Autodesk Fusion 360 part; units mm, degrees
sketch "Sketch1" plane through (0, 0, 0) normal (1, 0, 0) x (0, 1, 0)
  line L0 (0, 0) -> (-230, 0)
  line L1 (-230, 0) -> (-230, 150)
  line L2 (-230, 150) -> (0, 150)
  line L3 (0, 150) -> (0, 0)
  line L4 (-230, 0) -> (-220, 0)
  line L5 (-220, 0) -> (-220, 150)
  line L6 (-220, 150) -> (-230, 150)
  line L7 (-230, 150) -> (-230, 0)
  dimension "d1" = 230
  dimension "d2" = 150
  dimension "d3" = 10
  dimension "d4" = 150
extrude "Extrude1" add sketch "Sketch1" against normal blind 10
extrude "Extrude2" add 1 faces at (-6.6667, -230, 50) along direction (0, -1, 0) blind 20
extrude "Extrude3" add 1 faces at (-6.6667, 0, 100) along direction (0, 1, 0) blind 20
sketch "Sketch2" plane through (0, 0, 0) normal (1, 0, 0) x (0, 1, 0)
  line L0 (20, 150) -> (-250, 150)
  line L1 (-250, 150) -> (-250, 0)
  line L2 (-250, 0) -> (20, 0)
  line L3 (20, 0) -> (20, 150)
  line L4 (-250, 0) -> (-240, 0)
  line L5 (-240, 0) -> (-240, 15)
  line L6 (-240, 15) -> (-250, 15)
  line L7 (-250, 15) -> (-250, 0)
  line L8 (0, 0) -> (-10, 0)
  line L9 (-10, 0) -> (-10, 15)
  line L10 (-10, 15) -> (0, 15)
  line L11 (0, 15) -> (0, 0)
  dimension "d11" = 10
  dimension "d12" = 15
  dimension "d13" = 10
  dimension "d14" = 15
  dimension "d46" = 230
extrude "Extrude12" add 1 faces at (-6.6667, -250, 50) along direction (0, -1, 0) blind 20
extrude "Extrude4" cut sketch "Sketch2" against normal blind 140 contours L1 L2 L4 L5 L6 L7 | L2 L8 L9 L10 L11
fillet "Fillet2" radius 20 1 edges at (-5, 20, 150)
sketch "Sketch3" plane through (0, 0, 0) normal (1, 0, 0) x (0, 1, 0)
  arc A0 (20, 130) -> (0, 150) centre (0, 130) ccw
  line L0 (0, 150) -> (-270, 150)
  line L1 (-250, 15) -> (-240, 15)
  line L2 (-240, 15) -> (-240, 0)
  line L3 (-270, 0) -> (-250, 0)
  line L4 (-10, 0) -> (-10, 15)
  line L5 (-10, 15) -> (0, 15)
  line L6 (0, 15) -> (0, 0)
  line L7 (0, 0) -> (20, 0)
  line L8 (20, 0) -> (20, 130)
  line L9 (-200, 0) -> (-30, 0)
  line L10 (-30, 0) -> (-30, 130)
  line L11 (-30, 130) -> (-200, 130)
  line L12 (-200, 130) -> (-200, 0)
  line L13 (-270, 150) -> (-270, 0)
  line L14 (-250, 0) -> (-250, 15)
  line L15 (-240, 0) -> (-10, 0)
extrude "Extrude5" cut sketch "Sketch3" against normal blind 100 contours L9 L10 L11 L12 L15
sketch "Sketch4" plane through (0, 0, 150) normal (0, 0, 1) x (-1, 0, 0)
  line L0 (0, 0) -> (10, 0)
  line L1 (10, 0) -> (10, 270)
  line L2 (0, 270) -> (0, 0)
  line L3 (0, 140) -> (-30, 140)
  line L4 (-30, 140) -> (-30, 111)
  line L5 (-30, 111) -> (0, 111)
  line L6 (0, 111) -> (0, 140)
  line L7 (0, 140) -> (-30, 111)
  line L8 (-30, 140) -> (0, 111)
  line L9 (-2, 138) -> (-28, 138)
  line L10 (-28, 138) -> (-28, 113)
  line L11 (-28, 113) -> (-2, 113)
  line L12 (-2, 113) -> (-2, 138)
  line L13 (-2, 138) -> (-28, 113) construction
  line L14 (-28, 138) -> (-2, 113) construction
  line L15 (10, 270) -> (0, 270)
  point P0 (-15, 125.5)
  dimension "d23" = 30
  dimension "d24" = 29
  dimension "d25" = 26
  dimension "d26" = 25
extrude "Extrude6" add sketch "Sketch4" against normal blind 10 contours L2 L6 L7 L8 L9 L11 L12 | L5 L7 L8 L11 | L3 L7 L8 L9 | L4 L7 L8 L9 L10 L11 | L7 L8 L11 | L7 L8 L9 L11 L12 | L7 L8 L9 | L7 L8 L9 L10 L11
extrude "Extrude7" cut sketch "Sketch4" against normal blind 8 contours L7 L8 L11 | L7 L8 L9 L11 L12 | L7 L8 L9 | L7 L8 L9 L10 L11
extrude "Extrude9" add 1 faces at (20, -120.6667, 140) along direction (0, 0, -1) blind 1
sketch "Sketch5" plane through (0, 0, 139) normal (0, 0, -1) x (1, 0, 0)
  line L0 (0, 140) -> (0, 111)
  line L1 (0, 111) -> (30, 111)
  line L2 (30, 111) -> (30, 140)
  line L3 (30, 140) -> (0, 140)
  circle A0 centre (13.026, 125.5717) radius 4
  line L4 (0, 111) -> (30, 111)
  line L5 (30, 111) -> (30, 140)
  line L6 (30, 140) -> (0, 140)
  line L7 (0, 140) -> (0, 111)
  line L8 (0, 126.0602) -> (5.9, 126.0602)
  line L9 (15.4722, 111) -> (15.4722, 119.2)
  line L10 (30, 125.5) -> (20.7, 125.5)
  line L11 (15, 140) -> (15, 131.8)
  line L12 (5.9, 119.2) -> (20.7, 119.2)
  line L13 (20.7, 119.2) -> (20.7, 131.8)
  line L14 (20.7, 131.8) -> (5.9, 131.8)
  line L15 (5.9, 131.8) -> (5.9, 119.2)
  dimension "d35" = 8
  dimension "d84" = 5.9
  dimension "d85" = 8.2
  dimension "d86" = 9.3
  dimension "d87" = 8.2
extrude "Extrude10" cut sketch "Sketch5" against normal blind 30 contours A0
fillet "Fillet3" radius 1.5 2 edges at (30, -111, 144.5) (30, -140, 144.5)
fillet "Fillet4" radius 3.5 1 edges at (0, -111, 144.5)
fillet "Fillet5" radius 3.5 1 edges at (0, -140, 144.5)
extrude "Extrude8" cut 1 faces at (24.342, -125.5239, 142) along direction (0, 0, -1) blind 1
fillet "Fillet7" radius 20 1 edges at (-5, -270, 150)
extrude "Extrude13" cut 1 faces at (-6.6667, -200, 86.6667) along direction (0, -1, 0) blind 20
fillet "Fillet8" radius 10 2 edges at (-5, -220, 130) (-5, -30, 130)
sketch "Sketch6" plane through (0, 0, 0) normal (1, 0, 0) x (0, 1, 0)
  line L0 (-210, 130) -> (-40, 130)
  arc A0 (-30, 120) -> (-40, 130) centre (-40, 120) ccw
  line L1 (-30, 120) -> (-30, 0)
  line L2 (-30, 0) -> (-10, 0)
  line L3 (-10, 0) -> (-10, 15)
  line L4 (-10, 15) -> (0, 15)
  line L5 (0, 15) -> (0, 0)
  line L6 (0, 0) -> (20, 0)
  line L7 (20, 0) -> (20, 130)
  arc A1 (20, 130) -> (0, 150) centre (0, 130) ccw
  line L8 (0, 150) -> (-107.5, 150)
  line L9 (-107.5, 150) -> (-107.5, 139)
  line L10 (-107.5, 139) -> (-143.5, 139)
  line L11 (-143.5, 139) -> (-143.5, 150)
  line L12 (-143.5, 150) -> (-250, 150)
  arc A2 (-250, 150) -> (-270, 130) centre (-250, 130) ccw
  line L13 (-270, 130) -> (-270, 0)
  line L14 (-270, 0) -> (-250, 0)
  line L15 (-250, 0) -> (-250, 15)
  line L16 (-250, 15) -> (-240, 15)
  line L17 (-240, 15) -> (-240, 0)
  line L18 (-240, 0) -> (-220, 0)
  line L19 (-220, 0) -> (-220, 120)
  arc A3 (-210, 130) -> (-220, 120) centre (-210, 120) ccw
  line L20 (-270, 0) -> (-198, 0)
  line L21 (-198, 0) -> (-198, 167.8427)
  line L22 (-198, 167.8427) -> (-270, 167.8427)
  line L23 (-270, 167.8427) -> (-270, 0)
  line L24 (20, 0) -> (-52, 0)
  line L25 (-52, 0) -> (-52, 156.7227)
  line L26 (-52, 156.7227) -> (20, 156.7227)
  line L27 (20, 156.7227) -> (20, 0)
  dimension "d57" = 72
extrude "Extrude14" cut sketch "Sketch6" against normal blind 180 contours L0 L12 A2 L13 L14 L15 L16 L17 L18 L19 A3 L20 L21 L23 | L0 L19 A3 L20 L21 | L0 A0 L1 L2 L3 L4 L5 L6 L7 A1 L8 L24 L25 L27 | L0 A0 L1 L24 L25 | L12 A2 L21 L22 L23 | A1 L8 L25 L26 L27
sketch "Sketch7" plane through (0, 0, 0) normal (1, 0, 0) x (0, 1, 0)
  line L0 (-198, 150) -> (-198, 130)
  line L1 (-198, 130) -> (-52, 130)
  line L2 (-52, 130) -> (-52, 150)
  line L3 (-52, 150) -> (-107.5, 150)
  line L4 (-107.5, 150) -> (-107.5, 139)
  line L5 (-107.5, 139) -> (-143.5, 139)
  line L6 (-143.5, 139) -> (-143.5, 150)
  line L7 (-143.5, 150) -> (-198, 150)
  line L8 (-198, 150) -> (-250, 150)
  line L9 (-52, 150) -> (0, 150)
  line L10 (-250, 150) -> (-250, 130)
  line L11 (-250, 130) -> (-198, 130)
  line L12 (0, 150) -> (0, 130)
  line L13 (0, 130) -> (-52, 130)
  dimension "d60" = 52
  dimension "d61" = 52
extrude "Extrude15" add sketch "Sketch7" against normal blind 10 contours L0 L8 L10 L11 | L2 L9 L12 L13
sketch "Sketch8" plane through (0, -250, 0) normal (0, -1, 0) x (1, 0, 0)
  line L0 (0, 130) -> (0, 150)
  line L1 (0, 150) -> (-10, 150)
  line L2 (-10, 150) -> (-10, 130)
  line L3 (-10, 130) -> (0, 130)
  circle A0 centre (-5, 140) radius 3.5
  dimension "d64" = 7
extrude "Extrude16" cut sketch "Sketch8" against normal blind 20 contours A0
sketch "Sketch9" plane through (0, 0, 0) normal (0, 1, 0) x (-1, 0, 0)
  line L0 (0, 150) -> (0, 130)
  line L1 (0, 130) -> (10, 130)
  line L2 (10, 130) -> (10, 150)
  line L3 (10, 150) -> (0, 150)
  circle A0 centre (5, 140) radius 3.5
  dimension "d67" = 7
extrude "Extrude17" cut sketch "Sketch9" against normal blind 20 contours A0
thread "Thread1"
thread "Thread2"
extrude "Extrude18" cut 1 faces at (-4.9128, -250, 147.8301) along direction (0, 1, 0) blind 15
extrude "Extrude19" cut 1 faces at (-4.9128, 0, 147.8301) along direction (0, -1, 0) blind 15
extrude "Extrude20" cut 1 faces at (-4.9128, -235, 147.8301) along direction (0, 1, 0) blind 50
extrude "Extrude21" cut 1 faces at (-3.9973, -230, 138.825) along direction (0, 1, 0) blind 59
extrude "Extrude22" cut 1 faces at (-4.9128, -15, 147.8301) along direction (0, -1, 0) blind 50
extrude "Extrude23" cut 1 faces at (-6.0027, -20, 138.825) along direction (0, -1, 0) blind 57
extrude "Extrude24" add 1 faces at (-3.9973, -171, 138.825) along direction (0, -1, 0) blind 2
thread "Thread3"
thread "Thread4"
sketch "Sketch10" plane through (0, 0, 150) normal (0, 0, 1) x (-1, 0, 0)
  line L0 (-28, 138) -> (-2, 138)
  line L1 (-2, 138) -> (-2, 113)
  line L2 (-2, 113) -> (-28, 113)
  line L3 (-28, 113) -> (-28, 138)
  line L4 (0, 65) -> (10, 65)
  line L5 (10, 65) -> (10, 185)
  line L6 (10, 185) -> (0, 185)
  line L7 (0, 185) -> (0, 143.5)
  arc A0 (-3.5, 140) -> (0, 143.5) centre (-3.5, 143.5) ccw
  line L8 (-3.5, 140) -> (-28.5, 140)
  arc A1 (-28.5, 140) -> (-30, 138.5) centre (-28.5, 138.5) ccw
  line L9 (-30, 138.5) -> (-30, 112.5)
  arc A2 (-30, 112.5) -> (-28.5, 111) centre (-28.5, 112.5) ccw
  line L10 (-28.5, 111) -> (-3.5, 111)
  arc A3 (0, 107.5) -> (-3.5, 111) centre (-3.5, 107.5) ccw
  line L11 (0, 107.5) -> (0, 65)
  line L12 (-2, 117.3316) -> (10, 117.3316)
  line L13 (10, 117.3316) -> (10, 136.568)
  line L14 (10, 136.568) -> (-2, 136.568)
  line L15 (-2, 136.568) -> (-2, 117.3316)
extrude "Extrude25" cut sketch "Sketch10" against normal blind 8 contours L1 L5 L12 L13 L14 L15
Design review of the part built by this model. Coordinates are the model's own, in mm. A direction names the side the tool comes from. Round coordinates to 2 decimals unless told otherwise and drop trailing zeros. Write each loop counter-clockwise with the first axis right and the second up, starting at its lowest first coordinate (ties: lowest second). Pieces come first, ordered by that corner, then holes. Notation, with made-up numbers: (7, 39.25) -> (21, 39.25) arc R17 ccw to (21, 62.25) -> close; hole circle Ø4 at (88, 75). An arc over 180 degrees is marked (long way). Answer in a Markdown table with one row per item.
Q1. Take a section at A-A, the plane x = 16. State the section outline as (y, z) points.
The answers:
| item | result |
|---|---|
| outline | (-140, 139) -> (-128.25, 139) -> (-128.25, 141) -> (-138, 141) -> (-138, 150) -> (-140, 150) -> close; (-122.9, 139) -> (-111, 139) -> (-111, 150) -> (-113, 150) -> (-113, 141) -> (-122.9, 141) -> close |
Q2. To check wall thickness, follow L1, parallel to Z at x = -5, y = -175; L2, parallel to Y at x = 21.5, z = 144.5; L3, parallel to X at y = -181.5, z = 140. State the ranges of each line that lie inside material, in increasing order. Write a range as [from, to].
The answers:
| item | result |
|---|---|
| L1 | [130, 136.5], [143.5, 150] |
| L2 | [-140, -138], [-113, -111] |
| L3 | [-10, -8.5], [-1.5, 0] |
Q3. For faces 4 (the face through (-4, -127, 142)), 5 (the face through (19, -126, 139)), 6 (the face through (16, -111, 145)), 7 (the face through (15, -138, 146)), list the 3-axis set-ups (+Z, -Z, +X, -X, +Y, -Y) from which the entire face can be reached by the end or side of a thin tool; tool diameter is ignored.
The answers:
| item | result |
|---|---|
| face 4 | +Z, -X |
| face 5 | -Z, +X, +Y, -Y |
| face 6 | +Z, -Z, +X, +Y |
| face 7 | +Z |
Q4. Draft analysis for pull direction Y (two halves, no side actions). For faces 1 (the face through (2, -119.89, 141.85)), 2 (the face through (-5, -173, 140)), 3 (the face through (-4.241, -70.916, 136.583)), state which applies: +Y half, -Y half, draft (parallel to the pull), parting line (faces both ways), or undercut.
The answers:
| item | result |
|---|---|
| face 1 | undercut |
| face 2 | -Y half |
| face 3 | draft |
Q5. Take a section at B-B, the plane x = -5. State the section outline as (y, z) points.
The answers:
| item | result |
|---|---|
| outline | (-185, 130) -> (-65, 130) -> (-65, 136.5) -> (-77, 136.5) -> (-77, 143.5) -> (-65, 143.5) -> (-65, 150) -> (-117.33, 150) -> (-117.33, 142) -> (-136.57, 142) -> (-136.57, 150) -> (-185, 150) -> (-185, 143.5) -> (-173, 143.5) -> (-173, 136.5) -> (-185, 136.5) -> close |
Q6. Take a section at C-C, the plane z = 146.25. State the section outline as (x, y) points, then the cut area to 3 significant figures.
The answers:
| item | result |
|---|---|
| outline | (-10, -185) -> (0, -185) -> (0, -143.5) arc R3.5 cw to (3.5, -140) -> (28.5, -140) arc R1.5 ccw to (30, -138.5) -> (30, -112.5) arc R1.5 ccw to (28.5, -111) -> (3.5, -111) arc R3.5 cw to (0, -107.5) -> (0, -65) -> (-10, -65) -> (-10, -117.33) -> (2, -117.33) -> (2, -113) -> (28, -113) -> (28, -138) -> (2, -138) -> (2, -136.57) -> (-10, -136.57) -> close |
| area | 1,190 mm² |
Q7. Take a section at D-D, the plane y = -81.5. State the section outline as (x, z) points, then the cut area to 3 significant figures.
The answers:
| item | result |
|---|---|
| outline | (-10, 130) -> (0, 130) -> (0, 150) -> (-10, 150) -> close |
| area | 200 mm² |
Q8. Clearance check with flat-ended pins moving along their axes: pin 1 Ø3.5 at (x, y) = (-2.5, -131) entering from +Z; pin 2 Ø4.5 at (x, z) = (13.5, 146) entering from +Y; pin 3 Ø13 at (x, y) = (13.03, -125.57) entering from -Z; pin 4 Ø8 at (x, z) = (-5, 140) entering from -Y. State where each tip first meets the part, or that it passes through.
The answers:
| item | result |
|---|---|
| pin 1 | z = 142 |
| pin 2 | y = -111 |
| pin 3 | z = 139 |
| pin 4 | y = -185 |
